Verification items for the finished model (mm, model axes). Face numbers are marked on the shaded views. Give positions to 0.01 mm unless a question says otherwise; leave off trailing zeros. Write each loop counter-clockwise with the first axis right and the second up, starting at its lowest first coordinate (ties: lowest second). Pieces come first, ordered by that corner, then holes.
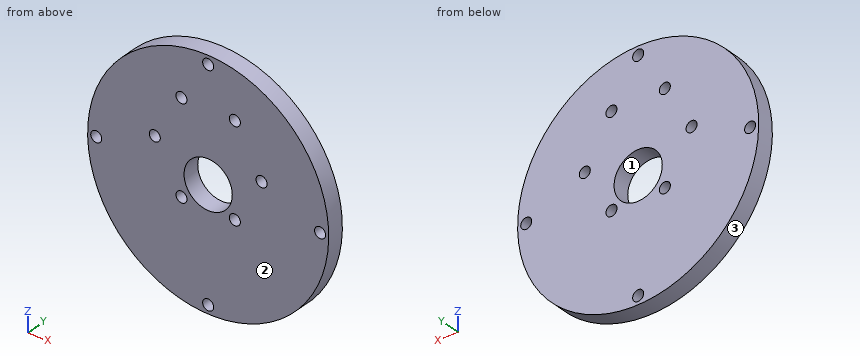
from build123d import *

# Parameters (mm, degrees)
SKETCH_1_R          = 35
EXTRUDE_1_DEPTH     = 5
SKETCH_3_R          = 1.6
CUT_EXTRUDE_1_DEPTH = 50.749371855
SKETCH_4_R          = 7
SKETCH_4_R_2        = 1.6
CUT_EXTRUDE_2_DEPTH = 50.749371855


with BuildPart() as part:
    # ｽｹｯﾁ1 → ﾎﾞｽ - 押し出し1 (new body)
    with BuildSketch(Plane(origin=(0, 0, 0), x_dir=(1, 0, 0), z_dir=(0, 1, 0))):
        with Locations(Location((0, 0, 0), (0, 0, 270))):
            Circle(SKETCH_1_R)
    extrude(amount=EXTRUDE_1_DEPTH)

    # ｽｹｯﾁ3 → ｶｯﾄ - 押し出し1 (cut, through all)
    with BuildSketch(Plane(origin=(0, 5, 0), x_dir=(1, 0, 0), z_dir=(0, 1, 0))):
        with Locations(Location((-32.5, 0, 0), (0, 0, 270))):
            Circle(SKETCH_3_R)
        with Locations(Location((0, 32.5, 0), (0, 0, 270))):
            Circle(SKETCH_3_R)
        with Locations(Location((32.5, 0, 0), (0, 0, 270))):
            Circle(SKETCH_3_R)
        with Locations(Location((0, -32.5, 0), (0, 0, 270))):
            Circle(SKETCH_3_R)
    extrude(amount=-CUT_EXTRUDE_1_DEPTH, mode=Mode.SUBTRACT)

    # ｽｹｯﾁ4 → ｶｯﾄ - 押し出し2 (cut, through all)
    with BuildSketch(Plane(origin=(0, 5, 0), x_dir=(1, 0, 0), z_dir=(0, 1, 0))):
        with Locations(Location((0, 0, 0), (0, 0, 270))):
            Circle(SKETCH_4_R)
        with Locations(Location((-15.5, -7, 0), (0, 0, 270))):
            Circle(SKETCH_4_R_2)
        with Locations(Location((-7.75, 6.423393759, 0), (0, 0, 270))):
            Circle(SKETCH_4_R_2)
        with Locations(Location((7.75, 6.423393759, 0), (0, 0, 270))):
            Circle(SKETCH_4_R_2)
        with Locations(Location((15.5, -7, 0), (0, 0, 270))):
            Circle(SKETCH_4_R_2)
        with Locations(Location((7.75, -20.423393759, 0), (0, 0, 270))):
            Circle(SKETCH_4_R_2)
        with Locations(Location((-7.75, -20.423393759, 0), (0, 0, 270))):
            Circle(SKETCH_4_R_2)
    extrude(amount=-CUT_EXTRUDE_2_DEPTH, mode=Mode.SUBTRACT)


solid = part.part
Item 1: Release check for a two-part mould opening along X. For the marked faces 1, 2 and 3 record: released by +X, released by -X, zero draft, split by the parting line, or undercut.
Answer key:
face 1: undercut
face 2: zero draft
face 3: split by the parting line
Item 2: Sectioned sample at C-C on z = -32.5. Record the cut outline in (x, y), then the cut area to 3 significant figures.
Answer key:
outline: (-12.99, 0) - (-1.6, 0) - (-1.6, 5) - (-12.99, 5) - close; (1.6, 0) - (12.99, 0) - (12.99, 5) - (1.6, 5) - close
area: 114 mm2
Item 3: Sectioned sample at B-B on y = 0.75. State how many separate pieces and enclosed holes the cut face has, then the cut area to 3 significant figures.
Answer key:
separate pieces: 1
enclosed holes: 11
area: 3,610 mm2
Item 4: Sectioned sample at A-A on x = 0. Record the cut outline in (y, z).
Answer key:
outline: (0, -35) - (5, -35) - (5, -34.1) - (0, -34.1) - close; (0, -30.9) - (5, -30.9) - (5, -7) - (0, -7) - close; (0, 7) - (5, 7) - (5, 30.9) - (0, 30.9) - close; (0, 34.1) - (5, 34.1) - (5, 35) - (0, 35) - close
Item 5: Sectioned sample at D-D on x = -15.5. Record the cut outline in (y, z).
Answer key:
outline: (0, -31.38) - (5, -31.38) - (5, 5.4) - (0, 5.4) - close; (0, 8.6) - (5, 8.6) - (5, 31.38) - (0, 31.38) - close
Item 6: Scan lines: line 1 along X through (y, z) = (2.35, 0); line 2 along X through (y, z) = (0.7, 19); line 3 along X through (y, z) = (2.4, -3). Record each from-to range of solid material in increasing order.
Answer key:
line 1: x = -35 to -34.1, -30.9 to -7, 7 to 30.9, 34.1 to 35
line 2: x = -29.39 to -8.48, -7.02 to 7.02, 8.48 to 29.39
line 3: x = -34.87 to -6.32, 6.32 to 34.87
Item 7: Depth check by flat-ended pin: pin 1 (1.5 mm diameter, centred on y = 2.5, z = -24.5, fed in from +X); pin 2 (3 mm diameter, centred on x = 11.5, y = 2.5, fed in from -Z); pin 3 (3 mm diameter, centred on x = 5, y = 1, fed in from +Z). Enter the tip coordinate at first touch or a pass-through.
Answer key:
pin 1: stops at x = 25.71
pin 2: stops at z = -33.54
pin 3: stops at z = 34.82
